```python
from build123d import *

# Parameters (mm, degrees)
F1_DEPTH = 25.4
F2_R     = 7.62


with BuildPart() as f1:
    # F0 (on Top) → F1 (new body)
    with BuildSketch(Plane.XY):
        Polygon((-44.45, 63.5), (-69.85, 63.5), (-69.85, 38.1), (-66.675, 38.1), (-66.675, 60.325), (-44.45, 60.325), align=None)
        Polygon((69.85, 63.5), (-44.45, 63.5), (-44.45, 60.325), (66.675, 60.325), (66.675, -60.325), (-66.675, -60.325), (-66.675, 38.1), (-69.85, 38.1), (-69.85, -63.5), (69.85, -63.5), align=None)
    extrude(amount=F1_DEPTH)

    # F2
    f2_edges = [f1.edges().sort_by_distance(p)[0] for p in [
        (66.675, 60.325, 12.7),
        (66.675, -60.325, 12.7),
        (-66.675, -60.325, 12.7),
        (-66.675, 60.325, 12.7),
    ]]
    fillet(f2_edges, radius=F2_R)


solid = f1.part
```
Could you check a few things on this model? Use its own coordinates, in mm. A direction names the side the tool comes from. Round coordinates to 2 decimals unless told otherwise and drop trailing zeros. Loops run counter-clockwise (first coordinate to the right, second up) from the corner with the lowest first, then second, coordinate; pieces in that order, holes last. Notation, with made-up numbers: (-7.75, 45.5) - (45.25, 45.5) arc R30 ccw to (45.25, 83.5) - close; hole circle Ø6 at (49, -21.75). An arc over 180 degrees is marked (long way). Answer in a Markdown table with one row per item. Add a question column.
(1) If we section it at C-C (z = 9): Please give me the cut outline in (x, y) (3 decimals).
(2) If we section it at A-A (y = -7): Please give me the cut outline in (x, z) (3 decimals), plus the area to 3 significant figures.
(3) If we section it at B-B (x = -1.5): Please give me the cut outline in (y, z) (3 decimals), plus the area to 3 significant figures.
(4) If we mould it in two halves opening along X, with no side actions, what happens to faces 1 (the face through (1, 63.5, 13)), 2 (the face through (69.85, -1, 13)), 3 (the face through (-66.675, -1, 13))? For each: pulls with the +X half, pulls with the -X half, needs draft (parallel to the pull), parting line crosses it, or undercut.
(5) For faces 4 (the face through (-6, -61, 25.4)), 5 (the face through (66.675, 1, 13)), which set-ups out of +Z, -Z, +X, -X, +Y, -Y let a thin tool reach every point of the face, with its end or its side?
(6) I need wall thicknesses on line 1 along X through (y, z) = (52.5, 9.5) (3 decimals); line 2 along Y through (x, z) = (35, 3.5) (3 decimals); line 3 along Y through (x, z) = (64, 16.5). Which ranges of each line are inside material? Lowest first, please.
Model answer:
| question | item | result |
|---|---|---|
| 1 | outline | (-69.85, -63.5) - (69.85, -63.5) - (69.85, 63.5) - (-69.85, 63.5) - close; hole (-66.675, -52.705) arc R7.62 ccw to (-59.055, -60.325) - (59.055, -60.325) arc R7.62 ccw to (66.675, -52.705) - (66.675, 52.705) arc R7.62 ccw to (59.055, 60.325) - (-59.055, 60.325) arc R7.62 ccw to (-66.675, 52.705) - close |
| 2 | outline | (-69.85, 0) - (-66.675, 0) - (-66.675, 25.4) - (-69.85, 25.4) - close; (66.675, 0) - (69.85, 0) - (69.85, 25.4) - (66.675, 25.4) - close |
| 2 | area | 161 mm² |
| 3 | outline | (-63.5, 0) - (-60.325, 0) - (-60.325, 25.4) - (-63.5, 25.4) - close; (60.325, 0) - (63.5, 0) - (63.5, 25.4) - (60.325, 25.4) - close |
| 3 | area | 161 mm² |
| 4 | face 1 | needs draft |
| 4 | face 2 | pulls with the +X half |
| 4 | face 3 | undercut |
| 5 | face 4 | +Z, +X, -X, +Y, -Y |
| 5 | face 5 | +Z, -Z |
| 6 | line 1 | x = -69.85 to -66.675, 66.675 to 69.85 |
| 6 | line 2 | y = -63.5 to -60.325, 60.325 to 63.5 |
| 6 | line 3 | y = -63.5 to -58.5, 58.5 to 63.5 |
